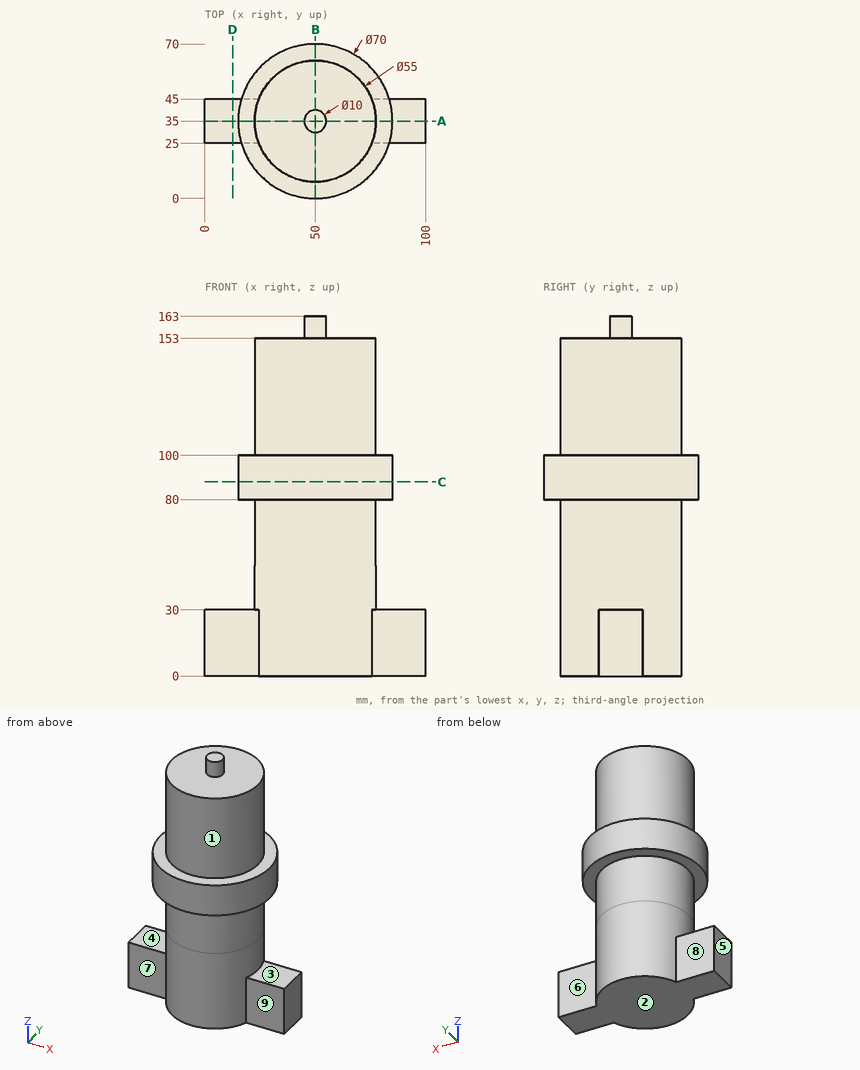
Study the drawing (mm; zero at the part's minimum x, y, z) and answer. A direction names the side the tool comes from. Round coordinates to 2 decimals unless told otherwise and drop trailing zeros. Loops run counter-clockwise (first coordinate to the right, second up) from the corner with the lowest first, then second, coordinate; pieces in that order, holes last. Notation, with made-up numbers: (30, 25) -> (71, 25) arc R35 ccw to (71, 58) -> close; hole circle Ø2 at (-2, 32). An arc over 180 degrees is marked (long way). Write each question's results on one line, items separated by ' | '. Start each with the question number.
1. For a pull along Z with two mould halves and no side action, classify the marked faces 1, 2, 3 and 4 as +Z half, -Z half, draft (parallel to the pull), parting line (faces both ways), or undercut.
2. Given pin 1 Ø19.5 at (x, z) = (8.5, 19) entering from -Y; pin 2 Ø12 at (x, y) = (45, 17.5) entering from +Z; pin 3 Ø1 at (x, z) = (27.5, 72) entering from -Y, each flat-ended and moving along its own axis, determine where each tip first touches the part or whether it passes through.
3. Find the intervals of material crossed by probe 1 along Z at (x, y) = (68, 52); probe 2 along Y at (x, z) = (17.5, 11); probe 3 along Z at (x, y) = (73.5, 53), in increasing order. Write a range as from..to.
4. Section D-D (x = 12.5) is taken. Determine the outline of the cut face in (y, z), plus the area to 3 significant figures.
5. A tool of negligible diameter and unlimited length cuts with its end or side. For the marked faces 5, 6, 7, 8 and 9, from which of +Z, -Z, +X, -X, +Y, -Y can it reach the whole face along a straight path? Write none if from no direction.
6. Section B-B (x = 50) is taken. Determine the outline of the cut face in (y, z), plus the area to 4 significant figures.
7. Section C-C (z = 88) is taken. Determine the outline of the cut face in (x, y), plus the area to 3 significant figures.
8. Section A-A (y = 35) is taken. Determine the outline of the cut face in (x, z).
Evaluation:
1) face 1: draft | face 2: -Z half | face 3: undercut | face 4: undercut
2) pin 1: stops at y = 25 | pin 2: stops at z = 153 | pin 3: stops at y = 18.5
3) probe 1: z = 0..153 | probe 2: y = 25..45 | probe 3: z = 80..100
4) outline: (25, 0) -> (45, 0) -> (45, 30) -> (25, 30) -> close | area: 600 mm2
5) face 5: +Z, -Z, -X, +Y, -Y | face 6: -Z, +X, +Y | face 7: -Z, -X, -Y | face 8: -Z, -X, +Y | face 9: -Z, +X, -Y
6) outline: (0, 80) -> (7.5, 80) -> (7.5, 0) -> (62.5, 0) -> (62.5, 80) -> (70, 80) -> (70, 100) -> (62.5, 100) -> (62.5, 153) -> (40, 153) -> (40, 163) -> (30, 163) -> (30, 153) -> (7.5, 153) -> (7.5, 100) -> (0, 100) -> close | area: 8,815 mm2
7) outline: circle Ø70 at (50, 35) | area: 3,850 mm2
8) outline: (0, 0) -> (100, 0) -> (100, 30) -> (77.5, 30) -> (77.5, 80) -> (85, 80) -> (85, 100) -> (77.5, 100) -> (77.5, 153) -> (55, 153) -> (55, 163) -> (45, 163) -> (45, 153) -> (22.5, 153) -> (22.5, 100) -> (15, 100) -> (15, 80) -> (22.5, 80) -> (22.5, 30) -> (0, 30) -> close
